from build123d import *

# Parameters (mm, degrees)
F0_R     = 12.7
F1_DEPTH = 60.325
F2_DEPTH = 19.05
F3_DEPTH = 19.05
F4_DEPTH = 25.4
F5_R     = 6.35
F5_W     = 50.881216
F5_H     = 22.3266
F6_DEPTH = 57.151


with BuildPart() as f1:
    # F0 (on Front) → F1 (new body)
    with BuildSketch(Plane.XZ):
        with BuildLine():
            Line((-91.8464, 0), (0, 0))
            Line((0, 0), (-5.9944, 22.352))
            Line((-5.9944, 22.352), (-66.405792, 22.352))
            ThreePointArc((-66.405792, 22.352), (-68.585221, 23.173417), (-69.680326, 25.22899))
            ThreePointArc((-69.680326, 25.22899), (-108.638041, 37.105058), (-91.8464, 0))
        make_face()
        with Locations((-91.8464, 22.352)):
            Circle(F0_R, mode=Mode.SUBTRACT)
        with BuildLine():
            Line((25.4, 22.352), (25.4, 0))
            Line((25.4, 0), (102.362, 0))
            Line((102.362, 0), (102.362, 14.478))
            ThreePointArc((102.362, 14.478), (100.055759, 20.045759), (94.488, 22.352))
            Line((94.488, 22.352), (61.5442, 22.352))
            Line((61.5442, 22.352), (58.2422, 22.352))
            Line((58.2422, 22.352), (39.1922, 22.352))
            Line((39.1922, 22.352), (25.4, 22.352))
        make_face()
        Polygon((-5.9944, 22.352), (0, 0), (25.4, 0), (25.4, 22.352), align=None)
    extrude(amount=-F1_DEPTH)

    # F0 (on Front) → F2 (join)
    with BuildSketch(Plane.XZ):
        with BuildLine():
            ThreePointArc((39.1922, 57.15), (35.618015, 38.434358), (25.4, 22.352))
            Line((25.4, 22.352), (39.1922, 22.352))
            Line((39.1922, 22.352), (58.2422, 22.352))
            Line((58.2422, 22.352), (61.5442, 22.352))
            ThreePointArc((61.5442, 22.352), (59.209333, 23.319133), (58.2422, 25.654))
            Line((58.2422, 25.654), (58.2422, 52.07))
            ThreePointArc((58.2422, 52.07), (56.754302, 55.662102), (53.1622, 57.15))
            Line((53.1622, 57.15), (39.1922, 57.15))
        make_face()
    extrude(amount=-F2_DEPTH)

    # F0 (on Front) → F3 (cut)
    with BuildSketch(Plane.XZ):
        Polygon((-5.9944, 22.352), (0, 0), (25.4, 0), (25.4, 22.352), align=None)
    extrude(amount=-F3_DEPTH, mode=Mode.SUBTRACT)

    # F0 (on Front) → F4 (cut)
    with BuildSketch(Plane.XZ):
        Polygon((-5.9944, 22.352), (0, 0), (25.4, 0), (25.4, 22.352), align=None)
    extrude(amount=-F4_DEPTH, mode=Mode.SUBTRACT)

    # F5 (on Top) → F6 (cut, through all)
    with BuildSketch(Plane.XY):
        with Locations((63.5, 37.973)):
            Circle(F5_R)
        with Locations((-91.8464, 30.1625)):
            Rectangle(F5_W, F5_H)
    extrude(amount=F6_DEPTH, mode=Mode.SUBTRACT)


solid = f1.part
Can you work these out from the model? Positions are in its coordinate system, mm. A direction names the side the tool comes from. Round coordinates to 2 decimals unless told otherwise and drop trailing zeros. Order: outer loops, then holes, each group sorted by start corner. A loop starts at its lowest first (then second) coordinate and runs counter-clockwise, first axis right, second up. Notation, with made-up numbers: M 33.25,-21.5 L 58.25,-21.5 A30 ccw 58.25,9.5 Z; hole C 11,75.5 d8. An arc over 180 degrees is marked long. Use a Markdown table: item, result.
1) If I drill on line 1 along Y through (x, z) = (63, 4) (3 decimals); line 2 along Z through (x, y) = (-16.5, 48); line 3 along Y through (x, z) = (37, 31), over which ranges is the centre line in solid material (lowest first)?
Geometry says:
| item | result |
|---|---|
| line 1 | y = 0 to 31.643, 44.303 to 60.325 |
| line 2 | z = 0 to 22.35 |
| line 3 | y = 0 to 19.05 |
2) Imagine slicing it at B-B (z = 29.5). List the corners of the cut face in (x, y) for me (3 decimals), then the cut area to 3 significant figures.
Geometry says:
| item | result |
|---|---|
| outline | M -113.025,0 L -102.344,0 L -102.344,18.999 L -113.025,18.999 Z; M -113.025,41.326 L -102.344,41.326 L -102.344,60.325 L -113.025,60.325 Z; M -81.349,0 L -70.668,0 L -70.668,18.999 L -81.349,18.999 Z; M -81.349,41.326 L -70.668,41.326 L -70.668,60.325 L -81.349,60.325 Z; M 31.007,0 L 58.242,0 L 58.242,19.05 L 31.007,19.05 Z |
| area | 1,330 mm² |
3) If we mould it in two halves opening along Z, with no side actions, what happens to faces 4 (the face through (-79.733, 50.692, 26.167)), 5 (the face through (-58, 0, 18)), 6 (the face through (-79.733, 9.367, 26.167)), 7 (the face through (-3.04, 12.52, 11.33))? For each: +Z half, -Z half, draft (parallel to the pull), parting line (faces both ways), or undercut.
Geometry says:
| item | result |
|---|---|
| face 4 | undercut |
| face 5 | draft |
| face 6 | undercut |
| face 7 | +Z half |
4) Imagine slicing it at C-C (z = 6). List the corners of the cut face in (x, y) for me (3 decimals).
Geometry says:
| item | result |
|---|---|
| outline | M -107.085,0 L -1.609,0 L -1.609,25.4 L 25.4,25.4 L 25.4,0 L 102.362,0 L 102.362,60.325 L -107.085,60.325 L -107.085,41.326 L -66.406,41.326 L -66.406,18.999 L -107.085,18.999 Z; hole C 63.5,37.973 d12.7 |
5) Imagine slicing it at D-D (x = 19). List the corners of the cut face in (y, z) for me (3 decimals).
Geometry says:
| item | result |
|---|---|
| outline | M 25.4,0 L 60.325,0 L 60.325,22.352 L 25.4,22.352 Z |
6) Imagine slicing it at A-A (x = 63.5). List the corners of the cut face in (y, z) for me (3 decimals), then the cut area to 3 significant figures.
Geometry says:
| item | result |
|---|---|
| outline | M 0,0 L 31.623,0 L 31.623,22.352 L 0,22.352 Z; M 44.323,0 L 60.325,0 L 60.325,22.352 L 44.323,22.352 Z |
| area | 1,060 mm² |
7) On a 3-axis mill with a long thin cutter (end or side, diameter ignored), from which of +Z, -Z, +X, -X, +Y, -Y can I reach the whole of each face in a straight line? I mean faces 1 (the face through (-66.406, 30, 11)), 2 (the face through (58.242, 9, 39)), 3 (the face through (47, 19.05, 40)). Say none if no direction works.
Geometry says:
| item | result |
|---|---|
| face 1 | +Z, -Z, -X |
| face 2 | +Z, +X, +Y, -Y |
| face 3 | +Z, +X, -X, +Y |
8) I'm going to push flat-ended pins straight in: P1, Ø21, axis at y = 5.5, z = 35.5, coming from the +X side; P2, Ø2, axis at x = 19, y = 36, coming from the +Z side; P3, Ø12, axis at y = 12.5, z = 37, coming from the -X side. Where does each tip first touch, or does it pass through?
Geometry says:
| item | result |
|---|---|
| P1 | stops at x = 58.31 |
| P2 | stops at z = 22.35 |
| P3 | stops at x = -112.46 |
